Could you check a few things on this drawing? It's one solid part, dimensions in mm from its lowest x, y, z. Round coordinates to 2 decimals unless told otherwise and drop trailing zeros. Write each loop counter-clockwise with the first axis right and the second up, starting at its lowest first coordinate (ties: lowest second). Pieces come first, ordered by that corner, then holes. Notation, with made-up numbers: (19, 81.25) - (67, 81.25) arc R21 cw to (67, 106.25) - close; hole circle Ø2 at (68.25, 60). An arc over 180 degrees is marked (long way). Put each result on its own line as item: value.
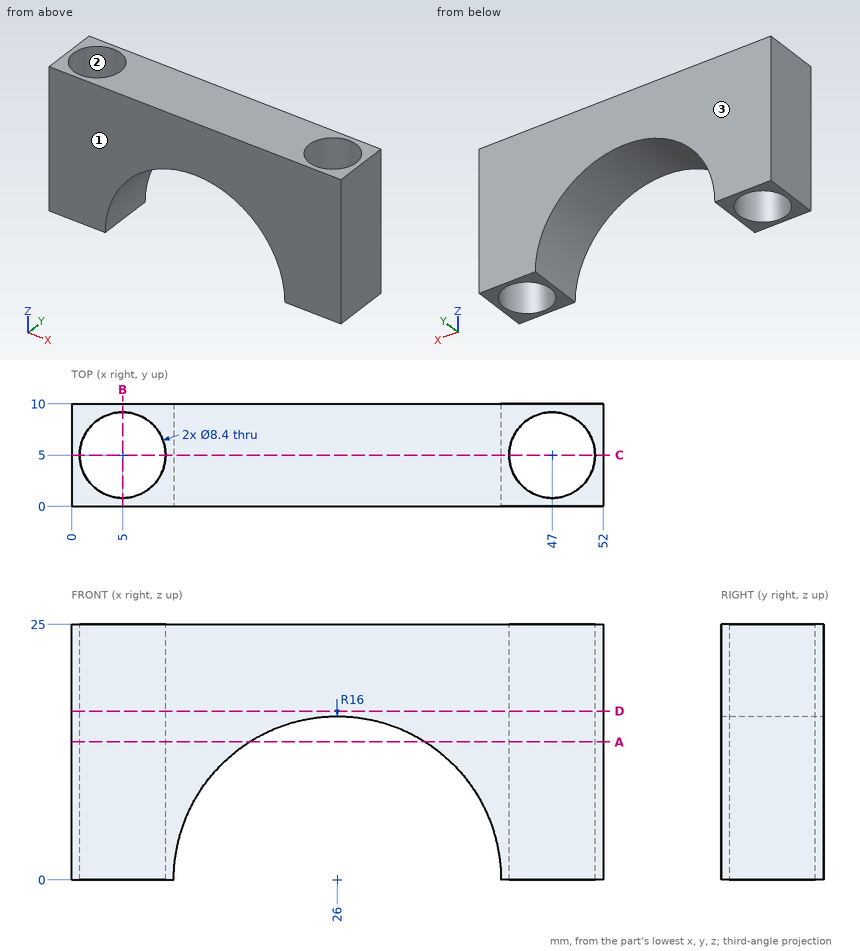
(1) If we mould it in two halves opening along Y, with no side actions, what happens to the marked faces 1, 2 and 3? For each: pulls with the +Y half, pulls with the -Y half, needs draft (parallel to the pull), parting line crosses it, or undercut.
Values found:
face 1: pulls with the -Y half
face 2: undercut
face 3: pulls with the +Y half
(2) Imagine slicing it at C-C, the plane y = 5. List the corners of the cut face in (x, z) for me, then the cut area to 3 significant figures.
Values found:
outline: (0, 0) - (0.8, 0) - (0.8, 25) - (0, 25) - close; (9.2, 0) - (10, 0) arc R16 cw to (42, 0) - (42.8, 0) - (42.8, 25) - (9.2, 25) - close; (51.2, 0) - (52, 0) - (52, 25) - (51.2, 25) - close
area: 478 mm^2
(3) Imagine slicing it at A-A, the plane z = 13.5. List the corners of the cut face in (x, y) for me, then the cut area to 3 significant figures.
Values found:
outline: (0, 0) - (17.41, 0) - (17.41, 10) - (0, 10) - close; (34.59, 0) - (52, 0) - (52, 10) - (34.59, 10) - close; hole circle Ø8.4 at (5, 5); hole circle Ø8.4 at (47, 5)
area: 237 mm^2
(4) I'm going to push a flat-ended pin straight in: pin 1 (5 mm diameter, centred on x = 5, y = 5, fed in from -Z). Where does the tip first touch, or does it pass through?
Values found:
pin 1: passes through
(5) Imagine slicing it at B-B, the plane x = 5. List the corners of the cut face in (y, z) for me.
Values found:
outline: (0, 0) - (0.8, 0) - (0.8, 25) - (0, 25) - close; (9.2, 0) - (10, 0) - (10, 25) - (9.2, 25) - close
(6) Please list where these lines run through material, in increasing order: probe 1 along X at (y, z) = (5, 18.5); probe 2 along X at (y, z) = (3.25, 13); probe 3 along X at (y, z) = (2.25, 16.25). Write a range as from..to.
Values found:
probe 1: x = 0..0.8, 9.2..42.8, 51.2..52
probe 2: x = 0..1.18, 8.82..16.67, 35.33..43.18, 50.82..52
probe 3: x = 0..1.83, 8.17..43.83, 50.17..52
(7) Imagine slicing it at D-D, the plane z = 16.5. List the corners of the cut face in (x, y) for me.
Values found:
outline: (0, 0) - (52, 0) - (52, 10) - (0, 10) - close; hole circle Ø8.4 at (5, 5); hole circle Ø8.4 at (47, 5)
